Source: CAD feature listing. Evaluate the final solid. Frame: model axes, mm. A direction names the side the tool comes from. Round coordinates to 2 decimals unless told otherwise and drop trailing zeros. Write each loop counter-clockwise with the first axis right and the second up, starting at its lowest first coordinate (ties: lowest second). Pieces come first, ordered by that corner, then holes. Notation, with made-up numbers: M -31.75,37 L 18.25,37 A17 cw 18.25,53 Z; hole C 8.5,53 d1. An arc over 180 degrees is marked long. Answer in a Markdown table with one row per item.
from build123d import *

# Parameters (mm, degrees)
SKETCH1_R           = 1.5
BOSS_EXTRUDE1_DEPTH = 3.5
BOSS_EXTRUDE2_DEPTH = 16
SKETCH4_R           = 13.5
BOSS_EXTRUDE3_DEPTH = 15
SKETCH5_R           = 23.5
BOSS_EXTRUDE4_DEPTH = 10
SKETCH6_W           = 10
SKETCH6_H           = 14
BOSS_EXTRUDE5_DEPTH = 20
SKETCH7_R           = 14
BOSS_EXTRUDE6_DEPTH = 15
CHAMFER1_SIZE       = 10
CUT_EXTRUDE4_REACH  = 91.925
SKETCH10_R          = 1.5
CHAMFER2_SIZE       = 5


with BuildPart() as part:
    # Sketch1 → Boss-Extrude1 (new body)
    with BuildSketch(Plane(origin=(0, 0, 0), x_dir=(1, 0, 0), z_dir=(0, 1, 0))):
        with BuildLine():
            Line((-50, -15), (-12.459935794, -15))
            ThreePointArc((-12.459935794, -15), (6.031468042, -18.543769661), (18.9, -4.8))
            ThreePointArc((18.9, -4.8), (19.537223284, -3.577601927), (20.653846154, -2.769230769))
            ThreePointArc((20.653846154, -2.769230769), (22.5, 0), (20.653846154, 2.769230769))
            ThreePointArc((20.653846154, 2.769230769), (19.537223284, 3.577601927), (18.9, 4.8))
            ThreePointArc((18.9, 4.8), (6.031468042, 18.543769661), (-12.459935794, 15))
            Line((-12.459935794, 15), (-50, 15))
            Line((-50, 15), (-50, -15))
        make_face()
        with Locations(Location((-30, -11.5, 0), (0, 0, 270))):
            Circle(SKETCH1_R, mode=Mode.SUBTRACT)
        with BuildLine():
            Line((-43, 8), (-17.783419244, 8))
            ThreePointArc((-17.783419244, 8), (-19.5, 0), (-17.783419244, -8))
            Line((-17.783419244, -8), (-43, -8))
            Line((-43, -8), (-43, 8))
        make_face(mode=Mode.SUBTRACT)
        with Locations(Location((-30, 11.5, 0), (0, 0, 270))):
            Circle(SKETCH1_R, mode=Mode.SUBTRACT)
        with Locations(Location((19.5, 0, 0), (0, 0, 270))):
            Circle(SKETCH1_R, mode=Mode.SUBTRACT)
    extrude(amount=BOSS_EXTRUDE1_DEPTH)

    # Sketch2 → Boss-Extrude2 (add)
    with BuildSketch(Plane.XY.offset(-8)):
        Polygon((-48, 3.5), (-48, 13.5), (-39, 29.088457268), (-35.535898385, 27.088457268), (-44, 12.42820323), (-44, 3.5), align=None)
    extrude(amount=BOSS_EXTRUDE2_DEPTH)

    # Sketch4 → Boss-Extrude3 (add)
    with BuildSketch(Plane(origin=(0, 3.5, 0), x_dir=(1, 0, 0), z_dir=(0, 1, 0))):
        with Locations(Location((0, 0, 0), (0, 0, 270))):
            Circle(SKETCH4_R)
    extrude(amount=BOSS_EXTRUDE3_DEPTH)

    # Sketch5 → Boss-Extrude4 (add)
    with BuildSketch(Plane(origin=(0, 18.5, 0), x_dir=(1, 0, 0), z_dir=(0, 1, 0))):
        with Locations(Location((0, 0, 0), (0, 0, 270))):
            Circle(SKETCH5_R)
    extrude(amount=BOSS_EXTRUDE4_DEPTH)

    # Sketch6 → Boss-Extrude5 (add)
    with BuildSketch(Plane(origin=(0, 28.5, 0), x_dir=(1, 0, 0), z_dir=(0, 1, 0))):
        with Locations((12, 0)):
            Rectangle(SKETCH6_W, SKETCH6_H)
    extrude(amount=BOSS_EXTRUDE5_DEPTH)

    # Sketch7 → Boss-Extrude6 (add)
    with BuildSketch(Plane(origin=(17, 0, 0), x_dir=(0, 0, -1), z_dir=(1, 0, 0))):
        with Locations((0, 55.5)):
            Circle(SKETCH7_R)
    extrude(amount=-BOSS_EXTRUDE6_DEPTH)

    # Chamfer1
    chamfer1_edges = [part.edges().sort_by_distance(p)[0] for p in [
        (0, 18.5, -13.5),
    ]]
    chamfer(chamfer1_edges, length=CHAMFER1_SIZE - 0.0001)  # a hair under: the kernel refuses the full size

    # Sketch10 → Cut-Extrude4 (cut, up to next)
    with BuildSketch(Plane.ZY.offset(-2), mode=Mode.PRIVATE) as cut_extrude4_sk1:
        with Locations((1.690473047, 59.125231148)):
            Circle(SKETCH10_R)
    cut_extrude4_tool1 = extrude(cut_extrude4_sk1.sketch, amount=-CUT_EXTRUDE4_REACH, mode=Mode.PRIVATE) & part.part
    # Sketch10 → Cut-Extrude4 (cut, up to next)
    with BuildSketch(Plane.ZY.offset(-2), mode=Mode.PRIVATE) as cut_extrude4_sk2:
        with Locations((-1.690473047, 51.874768852)):
            Circle(SKETCH10_R)
    cut_extrude4_tool2 = extrude(cut_extrude4_sk2.sketch, amount=-CUT_EXTRUDE4_REACH, mode=Mode.PRIVATE) & part.part
    add(cut_extrude4_tool1.solids().sort_by_distance((2, 59.125231, 1.690473))[0], mode=Mode.SUBTRACT)
    add(cut_extrude4_tool2.solids().sort_by_distance((2, 51.874769, -1.690473))[0], mode=Mode.SUBTRACT)

    # Chamfer2
    chamfer2_edges = [part.edges().sort_by_distance(p)[0] for p in [
        (7, 41.5, 0),
    ]]
    chamfer(chamfer2_edges, length=CHAMFER2_SIZE - 0.0001)  # a hair under: the kernel refuses the full size


solid = part.part
Q1. Section C-C (y = 25). Return loops of the section in (x, z), and give its area (3 significant figures).
Solutions:
| item | result |
|---|---|
| outline | M -41.36,-8 L -36.74,-8 L -36.74,8 L -41.36,8 Z; C 0,0 d47 |
| area | 1,810 mm2 |
Q2. Section D-D (y = 55.5). Return loops of the section in (x, z).
Solutions:
| item | result |
|---|---|
| outline | M 2,-14 L 17,-14 L 17,14 L 2,14 Z |
Q3. Contact query for flat-ended pins moving along their axis: pin 1 Ø6 at (y, z) = (35.5, 0.5) entering from +X; pin 2 Ø2 at (x, y) = (11, 38) entering from -Z; pin 3 Ø1 at (x, y) = (-33.5, 1) entering from +Z. Output: stop coordinate, or through.
Solutions:
| item | result |
|---|---|
| pin 1 | stops at x = 17 |
| pin 2 | stops at z = -7 |
| pin 3 | stops at z = 15 |
Q4. Access query for faces 1 (the cylindrical face through (6.292, 1.726, -18.457)), 2 (the flat face through (17, 49, 0)), 3 (the cylindrical face through (20.765, 1.726, 0.806)), 4 (the cylindrical face through (-13.18, 5.97, -2.93)). Directions: +Z, -Z, +X, -X, +Y, -Y. A direction counts if a zero-diameter tool reaches every point of the face in a straight line with its end or side. Return the directions, or none.
Solutions:
| item | result |
|---|---|
| face 1 | -Z, -Y |
| face 2 | +Z, -Z, +X, +Y |
| face 3 | -Y |
| face 4 | none |
Q5. Material intervals for probe 1 along X at (y, z) = (0.9, 11.5); probe 2 along Y at (x, z) = (13.5, 12.5); probe 3 along X at (y, z) = (34, -5), sorted ascending.
Solutions:
| item | result |
|---|---|
| probe 1 | x = -50 to -31.5, -28.5 to 15.75 |
| probe 2 | y = 0 to 3.5, 13.4 to 28.5, 49.2 to 61.8 |
| probe 3 | x = 7 to 17 |
Q6. Section A-A (x = -33). Return loops of the section in (y, z), and give its area (3 significant figures).
Solutions:
| item | result |
|---|---|
| outline | M 0,-15 L 3.5,-15 L 3.5,-8 L 0,-8 Z; M 0,8 L 3.5,8 L 3.5,15 L 0,15 Z |
| area | 49.0 mm2 |
Q7. Pull-direction query (X, two-part tool) for faces 5 (the flat face through (-43.56, 21.19, -0.11)), 6 (the flat face through (-31, 2, 15)), 7 (the flat face through (-39.71, 19.86, -0.11)); classes: pulls with the +X half, pulls with the -X half, needs draft (parallel to the pull), parting line crosses it, or undercut.
Solutions:
| item | result |
|---|---|
| face 5 | pulls with the -X half |
| face 6 | needs draft |
| face 7 | undercut |
